Could you check a few things on this model? Use its own coordinates, in mm. Face numbers are marked on the shaded views. A direction names the side the tool comes from. Round coordinates to 2 decimals unless told otherwise and drop trailing zeros. Loops run counter-clockwise (first coordinate to the right, second up) from the corner with the lowest first, then second, coordinate; pieces in that order, holes last. Notation, with made-up numbers: M 28,77 L 38,77 A17 cw 38,106 Z; hole C -40,-28.75 d5. An arc over 180 degrees is marked long. Answer in a Markdown table with one row per item.
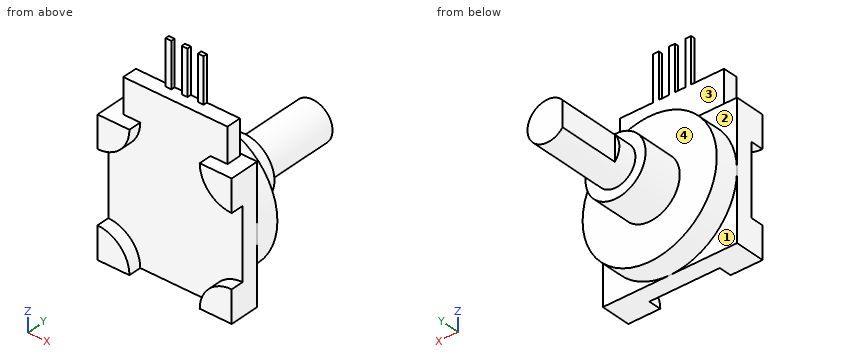
```python
from build123d import *

# Parameters (mm, degrees)
SKETCH1_W               = 21
SKETCH1_H               = 21
BOSS_EXTRUDE1_DEPTH     = 4.7
SKETCH2_R               = 10.5
BOSS_EXTRUDE2_DEPTH     = 3.73
SKETCH3_R               = 4.7
BOSS_EXTRUDE3_DEPTH     = 6.3
SKETCH4_R               = 3.1
BOSS_EXTRUDE4_DEPTH     = 12.6
CUT_EXTRUDE1_DEPTH      = 2
SKETCH6_W               = 16.3
SKETCH6_H               = 2.3
BOSS_EXTRUDE5_DEPTH     = 5.4
SKETCH7_W               = 5.95
SKETCH7_H               = 0.6
BOSS_EXTRUDE6_DEPTH     = 7
SKETCH8_W               = 1.625
SKETCH8_H               = 7
CUT_EXTRUDE2_DEPTH      = 24.03
CUT_EXTRUDE2_DEPTH_BACK = 5.3
CUT_EXTRUDE3_DEPTH      = 9.64


with BuildPart() as part:
    # Sketch1 → Boss-Extrude1 (new body)
    with BuildSketch(Plane(origin=(0, 0, 0), x_dir=(1, 0, 0), z_dir=(0, 1, 0))):
        with Locations((10.5, 10.5)):
            Rectangle(SKETCH1_W, SKETCH1_H)
    extrude(amount=BOSS_EXTRUDE1_DEPTH)

    # Sketch2 → Boss-Extrude2 (add)
    with BuildSketch(Plane(origin=(0, 4.7, 0), x_dir=(1, 0, 0), z_dir=(0, 1, 0))):
        with Locations((10.5, 10.5)):
            Circle(SKETCH2_R)
    extrude(amount=BOSS_EXTRUDE2_DEPTH)

    # Sketch3 → Boss-Extrude3 (add)
    with BuildSketch(Plane(origin=(0, 8.43, 0), x_dir=(1, 0, 0), z_dir=(0, 1, 0))):
        with Locations((10.5, 10.5)):
            Circle(SKETCH3_R)
    extrude(amount=BOSS_EXTRUDE3_DEPTH)

    # Sketch4 → Boss-Extrude4 (add)
    with BuildSketch(Plane(origin=(0, 14.73, 0), x_dir=(1, 0, 0), z_dir=(0, 1, 0))):
        with Locations((10.5, 10.5)):
            Circle(SKETCH4_R)
    extrude(amount=BOSS_EXTRUDE4_DEPTH)

    # Sketch5 → Cut-Extrude1 (cut)
    with BuildSketch(Plane.XZ):
        with BuildLine():
            Line((5, 0), (16, 0))
            ThreePointArc((16, 0), (17.464466094, -3.535533906), (21, -5))
            Line((21, -5), (21, -16))
            ThreePointArc((21, -16), (17.464466094, -17.464466094), (16, -21))
            Line((16, -21), (5, -21))
            ThreePointArc((5, -21), (3.535533906, -17.464466094), (0, -16))
            Line((0, -16), (0, -5))
            ThreePointArc((0, -5), (3.535533906, -3.535533906), (5, 0))
        make_face()
    extrude(amount=-CUT_EXTRUDE1_DEPTH, mode=Mode.SUBTRACT)

    # Sketch6 → Boss-Extrude5 (add)
    with BuildSketch(Plane.XY):
        with Locations((10.5, 3.15)):
            Rectangle(SKETCH6_W, SKETCH6_H)
    extrude(amount=BOSS_EXTRUDE5_DEPTH)

    # Sketch7 → Boss-Extrude6 (add)
    with BuildSketch(Plane.XY.offset(5.4)):
        with Locations((10.5, 4)):
            Rectangle(SKETCH7_W, SKETCH7_H)
    extrude(amount=BOSS_EXTRUDE6_DEPTH)

    # Sketch8 → Cut-Extrude2 (cut, two sides)
    with BuildSketch(Plane(origin=(0, 4.3, 0), x_dir=(1, 0, 0), z_dir=(0, 1, 0))) as cut_extrude2_sk:
        with Locations((9.2375, -8.9)):
            Rectangle(SKETCH8_W, SKETCH8_H)
        with Locations((11.7625, -8.9)):
            Rectangle(SKETCH8_W, SKETCH8_H)
    extrude(amount=CUT_EXTRUDE2_DEPTH, mode=Mode.SUBTRACT)
    extrude(cut_extrude2_sk.sketch, amount=-CUT_EXTRUDE2_DEPTH_BACK, mode=Mode.SUBTRACT)

    # Sketch9 → Cut-Extrude3 (cut)
    with BuildSketch(Plane(origin=(0, 27.33, 0), x_dir=(1, 0, 0), z_dir=(0, 1, 0))):
        with BuildLine():
            Line((8.1, 12.462141687), (8.1, 8.537858313))
            ThreePointArc((8.1, 8.537858313), (7.4, 10.5), (8.1, 12.462141687))
        make_face()
    extrude(amount=-CUT_EXTRUDE3_DEPTH, mode=Mode.SUBTRACT)


solid = part.part
```
1) I want a section at A-A, the plane z = 8. Please give me the cut outline in (x, y) (3 decimals), plus the area to 3 significant figures.
Computed:
| item | result |
|---|---|
| outline | M 7.525,3.7 L 8.425,3.7 L 8.425,4.3 L 7.525,4.3 Z; M 10.05,3.7 L 10.95,3.7 L 10.95,4.3 L 10.05,4.3 Z; M 12.575,3.7 L 13.475,3.7 L 13.475,4.3 L 12.575,4.3 Z |
| area | 1.62 mm² |
2) I need wall thicknesses on line 1 (Y direction, x = 16.5, z = -6.5); line 2 (Z direction, x = 16.25, y = 4.25); line 3 (Y direction, x = 20.25, z = -2.5). Which ranges of each line are inside material? Lowest first, please.
Computed:
| item | result |
|---|---|
| line 1 | y = 2 to 8.43 |
| line 2 | z = -21 to 5.4 |
| line 3 | y = 0 to 4.7 |
3) I want a section at D-D, the plane x = 1.75. Please give me the cut outline in (y, z), plus the area to 3 significant figures.
Computed:
| item | result |
|---|---|
| outline | M 0,-21 L 4.7,-21 L 4.7,-16.3 L 8.43,-16.3 L 8.43,-4.7 L 4.7,-4.7 L 4.7,0 L 0,0 L 0,-4.68 L 2,-4.68 L 2,-16.32 L 0,-16.32 Z |
| area | 119 mm² |
4) I want a section at B-B, the plane x = 16.75. Please give me the cut outline in (y, z).
Computed:
| item | result |
|---|---|
| outline | M 0,-21 L 4.7,-21 L 4.7,-18.94 L 8.43,-18.94 L 8.43,-2.06 L 4.7,-2.06 L 4.7,0 L 4.3,0 L 4.3,5.4 L 2,5.4 L 2,0 L 0,0 L 0,-2.63 L 2,-2.63 L 2,-18.37 L 0,-18.37 Z |
5) Will these pins go through, and if not, where does the flat tip stop? P1, Ø1, axis at x = 16.5, y = 12, coming from the -Z side; P2, Ø12, axis at y = 9, z = 5.5, coming from the -X side; P3, Ø8, axis at x = 11.5, y = 18.5, coming from the -Z side; P4, Ø0.7, axis at y = 4, z = 10.5, coming from the -X side (3 decimals).
Computed:
| item | result |
|---|---|
| P1 | passes through |
| P2 | stops at x = 2.35 |
| P3 | stops at z = -15.2 |
| P4 | stops at x = 7.525 |
6) Which directions (+Z, -Z, +X, -X, +Y, -Y) give clear straight access to the entire face, cutting with the end or side of a thin tool? Please do the marked faces 1, 2, 3 and 4.
Computed:
| item | result |
|---|---|
| face 1 | -Z, -X, +Y |
| face 2 | +Z, -X, +Y |
| face 3 | +Z, +X, -X, +Y |
| face 4 | +Y |
